Geometry: final body of the model. Coordinates: model frame, mm. Give positions to 0.01 mm unless a question says otherwise; leave off trailing zeros. Loops run counter-clockwise (first coordinate to the right, second up) from the corner with the lowest first, then second, coordinate; pieces in that order, holes last. Notation, with made-up numbers: (63.25, -10) -> (82.25, -10) arc R32 ccw to (82.25, 19) -> close; hole circle Ø7 at (-10.75, -14.5). An arc over 180 degrees is marked (long way). Answer in a Markdown table with one row per item. Add a question column.
from build123d import *

# Parameters (mm, degrees)
SKETCH1_W           = 60
SKETCH1_H           = 40
BOSS_EXTRUDE1_DEPTH = 5
SKETCH2_R           = 1.6
CUT_EXTRUDE1_DEPTH  = 5
FILLET1_R           = 1
FILLET2_R           = 1


with BuildPart() as part:
    # Sketch1 → Boss-Extrude1 (new body)
    with BuildSketch(Plane(origin=(0, 0, 0), x_dir=(1, 0, 0), z_dir=(0, 1, 0))):
        Rectangle(SKETCH1_W, SKETCH1_H)
    extrude(amount=BOSS_EXTRUDE1_DEPTH)

    # Sketch2 → Cut-Extrude1 (cut)
    with BuildSketch(Plane(origin=(0, 5, 0), x_dir=(1, 0, 0), z_dir=(0, 1, 0))):
        with Locations(Location((-25, 15, 0), (0, 0, 270))):
            Circle(SKETCH2_R)
        with Locations(Location((25, -15, 0), (0, 0, 270))):
            Circle(SKETCH2_R)
        with Locations(Location((-25, -15, 0), (0, 0, 270))):
            Circle(SKETCH2_R)
        with Locations(Location((25, 15, 0), (0, 0, 270))):
            Circle(SKETCH2_R)
    extrude(amount=-CUT_EXTRUDE1_DEPTH, mode=Mode.SUBTRACT)

    # Fillet1
    fillet1_edges = [part.edges().sort_by_distance(p)[0] for p in [
        (-30, 5, 0),
        (0, 5, 20),
        (30, 5, 0),
        (0, 5, -20),
    ]]
    fillet(fillet1_edges, radius=FILLET1_R)

    # Fillet2
    # the kernel refuses this fillet: 1 mm, written as the material it takes off along each edge
    with BuildSketch(Plane(origin=(29, 4, -19), x_dir=(1, 0, 0), z_dir=(0, 0, -1))) as fillet2_piece_1_section:
        Polygon((0, 0), (FILLET2_R, 0), (FILLET2_R, -FILLET2_R), (0, -FILLET2_R), align=None)
    fillet2_piece_1 = extrude(amount=FILLET2_R, mode=Mode.PRIVATE)
    fillet2_piece_1 = fillet2_piece_1 - Plane(origin=(29, 4, -19), x_dir=(-0.7071067811865475, -0.7071067811865475, 0), z_dir=(0, 0, -1)) * Sphere(FILLET2_R, mode=Mode.PRIVATE)
    add(fillet2_piece_1, mode=Mode.SUBTRACT)
    with BuildSketch(Plane(origin=(29, 4, 19), x_dir=(0, 0, 1), z_dir=(1, 0, 0))) as fillet2_piece_2_section:
        Polygon((0, 0), (FILLET2_R, 0), (FILLET2_R, -FILLET2_R), (0, -FILLET2_R), align=None)
    fillet2_piece_2 = extrude(amount=FILLET2_R, mode=Mode.PRIVATE)
    fillet2_piece_2 = fillet2_piece_2 - Plane(origin=(29, 4, 19), x_dir=(0, -0.7071067811865475, -0.7071067811865475), z_dir=(1, 0, 0)) * Sphere(FILLET2_R, mode=Mode.PRIVATE)
    add(fillet2_piece_2, mode=Mode.SUBTRACT)
    with BuildSketch(Plane(origin=(-29, 4, -19), x_dir=(-1, 0, 0), z_dir=(0, 0, -1))) as fillet2_piece_3_section:
        Polygon((0, 0), (FILLET2_R, 0), (FILLET2_R, FILLET2_R), (0, FILLET2_R), align=None)
    fillet2_piece_3 = extrude(amount=FILLET2_R, mode=Mode.PRIVATE)
    fillet2_piece_3 = fillet2_piece_3 - Plane(origin=(-29, 4, -19), x_dir=(0.7071067811865475, -0.7071067811865475, 0), z_dir=(0, 0, -1)) * Sphere(FILLET2_R, mode=Mode.PRIVATE)
    add(fillet2_piece_3, mode=Mode.SUBTRACT)
    with BuildSketch(Plane(origin=(-29, 4, 19), x_dir=(0, 0, 1), z_dir=(-1, 0, 0))) as fillet2_piece_4_section:
        Polygon((0, 0), (FILLET2_R, 0), (FILLET2_R, FILLET2_R), (0, FILLET2_R), align=None)
    fillet2_piece_4 = extrude(amount=FILLET2_R, mode=Mode.PRIVATE)
    fillet2_piece_4 = fillet2_piece_4 - Plane(origin=(-29, 4, 19), x_dir=(0, -0.7071067811865475, -0.7071067811865475), z_dir=(-1, 0, 0)) * Sphere(FILLET2_R, mode=Mode.PRIVATE)
    add(fillet2_piece_4, mode=Mode.SUBTRACT)
    with BuildSketch(Plane(origin=(-30, -2.5, 20), x_dir=(0, 0, -1), z_dir=(0, 1, 0)), Plane(origin=(-30, -2.5, -20), x_dir=(1, 0, 0), z_dir=(0, 1, 0))) as fillet2_piece_5:
        with BuildLine():
            CenterArc((FILLET2_R, -FILLET2_R), FILLET2_R, 90, 90)
            Line((0, -FILLET2_R), (0, 0))
            Line((0, 0), (FILLET2_R, 0))
        make_face()
    extrude(amount=6.5, mode=Mode.SUBTRACT)
    with BuildSketch(Plane(origin=(30, -2.5, -20), x_dir=(-1, 0, 0), z_dir=(0, 1, 0)), Plane(origin=(30, -2.5, 20), x_dir=(0, 0, -1), z_dir=(0, 1, 0))) as fillet2_piece_6:
        with BuildLine():
            CenterArc((FILLET2_R, FILLET2_R), FILLET2_R, 180, 90)
            Line((0, FILLET2_R), (0, 0))
            Line((0, 0), (FILLET2_R, 0))
        make_face()
    extrude(amount=6.5, mode=Mode.SUBTRACT)


solid = part.part
(1) Cut plane A-A on z = 15. Return the cut outline in (x, y), then the cut area to 3 significant figures.
(2) Draft query along X for faces 1 (the cylindrical face through (25.07, 2.54, 13.4)), 2 (the flat face through (30, 2, 0)), 3 (the flat face through (0, 0, 0)). Return one class per face: +X half, -X half, draft (parallel to the pull), parting line (faces both ways), or undercut.
(3) Material intervals for line 1 along X through (y, z) = (2.3, 15); line 2 along Z through (x, y) = (-24, 1.4); line 3 along X through (y, z) = (2.6, 16), sorted ascending. Write a range as from..to.
(4) Cut plane B-B on x = -25. Return the cut outline in (y, z).
Answer list:
| question | item | result |
|---|---|---|
| 1 | outline | (-30, 0) -> (-26.6, 0) -> (-26.6, 5) -> (-29, 5) arc R1 ccw to (-30, 4) -> close; (-23.4, 0) -> (23.4, 0) -> (23.4, 5) -> (-23.4, 5) -> close; (26.6, 0) -> (30, 0) -> (30, 4) arc R1 ccw to (29, 5) -> (26.6, 5) -> close |
| 1 | area | 268 mm² |
| 2 | face 1 | undercut |
| 2 | face 2 | +X half |
| 2 | face 3 | draft |
| 3 | line 1 | x = -30..-26.6, -23.4..23.4, 26.6..30 |
| 3 | line 2 | z = -20..-16.25, -13.75..13.75, 16.25..20 |
| 3 | line 3 | x = -30..-26.25, -23.75..23.75, 26.25..30 |
| 4 | outline | (0, -20) -> (4, -20) arc R1 ccw to (5, -19) -> (5, -16.6) -> (0, -16.6) -> close; (0, -13.4) -> (5, -13.4) -> (5, 13.4) -> (0, 13.4) -> close; (0, 16.6) -> (5, 16.6) -> (5, 19) arc R1 ccw to (4, 20) -> (0, 20) -> close |
